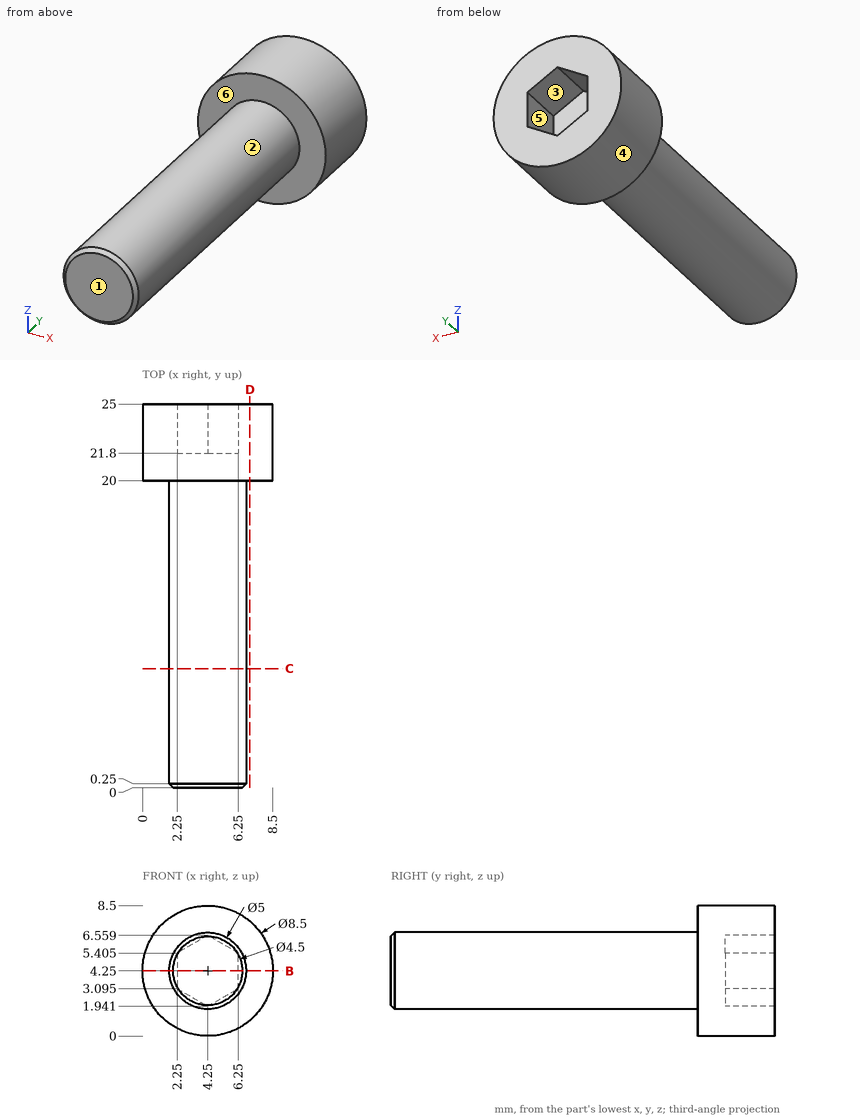
Design review of the part shown in the three views and the two pictorial views. Dimensions are in mm from the part's minimum x, y and z. A direction names the side the tool comes from. Round coordinates to 2 decimals unless told otherwise and drop trailing zeros. Write each loop counter-clockwise with the first axis right and the second up, starting at its lowest first coordinate (ties: lowest second). Pieces come first, ordered by that corner, then holes. Notation, with made-up numbers: (9, 48) - (14, 48) arc R20 ccw to (14, 70) - close; hole circle Ø2 at (-7.75, -23). An arc over 180 degrees is marked (long way). Return JSON: item names as keys, results as strings. Group by question number.
Item 1: The part is to be moulded in two halves that separate along Z. For the marked faces 1, 2 and 3, say which applies: pulls with the +Z half, pulls with the -Z half, needs draft (parallel to the pull), parting line crosses it, or undercut.
Item 2: Insertion check: P1, Ø1.5, axis at y = 11, z = 5.5, coming from the +X side; P2, Ø4, axis at x = 3, y = 13.5, coming from the +Z side; P3, Ø3, axis at x = 4, y = 11.5, coming from the -Z side. Each pin has a flat end and moves straight along its axis. Give the tip position at first contact, or say it passes through.
Item 3: Machinability: for the marked faces 4, 5 and 6, which of the approach directions +Z, -Z, +X, -X, +Y, -Y give a long, thin tool a straight path to every point of the face, cutting with its end or side? Answer none if there is none.
Item 4: We need section B-B on z = 4.25. Write out the cut boundary in (x, y), and give its area (3 significant figures).
Item 5: We need section D-D on x = 7. Write out the cut boundary in (y, z), and give its area (3 significant figures).
Item 6: We need section C-C on y = 7.75. Write out the cut boundary in (x, z), and give its area (3 significant figures).
Item 7: For probe 1 along Y at (x, z) = (6, 6.5); probe 2 along X at (y, z) = (23, 3) (1 decimal); probe 3 along X at (y, z) = (19.75, 2.75), list the stretches that pass through material, from the lowest coordinate up. Write a range as [from, to].
Model answer:
{
 "1": {"face 1": "needs draft", "face 2": "parting line crosses it", "face 3": "undercut"},
 "2": {"P1": "stops at x = 6.7", "P2": "stops at z = 6.75", "P3": "stops at z = 1.75"},
 "3": {"face 4": "+Y, -Y", "face 5": "+Y", "face 6": "-Y"},
 "4": {"outline": "(0, 20) - (1.75, 20) - (1.75, 0.25) - (2, 0) - (6.5, 0) - (6.75, 0.25) - (6.75, 20) - (8.5, 20) - (8.5, 25) - (6.25, 25) - (6.25, 21.8) - (2.25, 21.8) - (2.25, 25) - (0, 25) - close", "area": "130 mm²"},
 "5": {"outline": "(20, 1.01) - (25, 1.01) - (25, 7.49) - (20, 7.49) - close", "area": "32.4 mm²"},
 "6": {"outline": "circle Ø5 at (4.25, 4.25)", "area": "19.6 mm²"},
 "7": {"probe 1": "y = [20, 25]", "probe 2": "x = [0.2, 2.4], [6.1, 8.3]", "probe 3": "x = [2.25, 6.25]"}
}
